Autodesk Inventor part; units mm, degrees
ref_plane "YZ Plane" through (0, 0, 0) normal (1, 0, 0) x (0, 1, 0)
ref_plane "XZ Plane" through (0, 0, 0) normal (0, 1, 0) x (-1, 0, 0)
ref_plane "XY Plane" through (0, 0, 0) normal (0, 0, 1) x (1, 0, 0)
sketch "Sketch1" plane through (0, 0, 0) normal (0, 0, 1) x (1, 0, 0)
  line L0 (-18.15, -21.15) -> (18.15, -21.15)
  line L1 (21.15, -18.15) -> (21.15, 18.15)
  line L2 (18.15, 21.15) -> (-18.15, 21.15)
  line L3 (-21.15, 18.15) -> (-21.15, -18.15)
  line L4 (-21.15, -21.15) -> (21.15, 21.15) construction
  line L5 (21.15, -21.15) -> (-21.15, 21.15) construction
  line L6 (-21.15, 18.15) -> (-18.15, 21.15)
  line L7 (18.15, 21.15) -> (21.15, 18.15)
  line L8 (21.15, -18.15) -> (18.15, -21.15)
  line L9 (-18.15, -21.15) -> (-21.15, -18.15)
  line L10 (-15.5, -15.5) -> (15.5, -15.5) construction
  line L11 (15.5, -15.5) -> (15.5, 15.5) construction
  line L12 (15.5, 15.5) -> (-15.5, 15.5) construction
  line L13 (-15.5, 15.5) -> (-15.5, -15.5) construction
  line L14 (-15.5, -15.5) -> (15.5, 15.5) construction
  line L15 (15.5, -15.5) -> (-15.5, 15.5) construction
  circle A0 centre (-15.5, 15.5) radius 1.5
  circle A1 centre (15.5, 15.5) radius 1.5
  circle A2 centre (15.5, -15.5) radius 1.5
  circle A3 centre (-15.5, -15.5) radius 1.5
  point P0 (0, 0)
  dimension "d0" = 42.3
  dimension "d1" = 42.3
  dimension "d2" = 3
  dimension "d3" = 3
  dimension "d4" = 3
  dimension "d5" = 3
  dimension "d6" = 3
  dimension "d7" = 3
  dimension "d8" = 3
  dimension "d9" = 3
  dimension "d10" = 31
  dimension "d11" = 31
  dimension "d12" = 3
  dimension "d13" = 3
  dimension "d14" = 3
  dimension "d15" = 3
extrude "Extrusion1" add sketch "Sketch1" along normal mid plane 48
sketch "Sketch2" plane through (0, 0, 0) normal (0, 0, 1) x (1, 0, 0)
  circle A0 centre (-15.5, 15.5) radius 1.5
  circle A1 centre (15.5, 15.5) radius 1.5
  circle A2 centre (15.5, -15.5) radius 1.5
  circle A3 centre (-15.5, -15.5) radius 1.5
  point P0 (0, 0)
extrude "Extrusion2" add sketch "Sketch2" along normal mid plane 40
sketch "Sketch3" plane through (0, 0, 0) normal (0, 0, 1) x (1, 0, 0)
  line L0 (10.8431, -20.5) -> (-10.8431, -20.5)
  line L1 (-20.5, -10.8431) -> (-20.5, 10.8431)
  line L2 (-10.8431, 20.5) -> (10.8431, 20.5)
  line L3 (20.5, 10.8431) -> (20.5, -10.8431)
  line L4 (20.5, -20.5) -> (-20.5, 20.5) construction
  line L5 (-20.5, -20.5) -> (20.5, 20.5) construction
  line L6 (-19.3284, 13.6716) -> (-13.6716, 19.3284)
  line L7 (13.6716, 19.3284) -> (19.3284, 13.6716)
  line L8 (19.3284, -13.6716) -> (13.6716, -19.3284)
  line L9 (-13.6716, -19.3284) -> (-19.3284, -13.6716)
  arc A0 (-10.8431, 20.5) -> (-13.6716, 19.3284) centre (-10.8431, 16.5) ccw
  arc A1 (-19.3284, 13.6716) -> (-20.5, 10.8431) centre (-16.5, 10.8431) ccw
  arc A2 (13.6716, 19.3284) -> (10.8431, 20.5) centre (10.8431, 16.5) ccw
  arc A3 (20.5, 10.8431) -> (19.3284, 13.6716) centre (16.5, 10.8431) ccw
  arc A4 (19.3284, -13.6716) -> (20.5, -10.8431) centre (16.5, -10.8431) ccw
  arc A5 (10.8431, -20.5) -> (13.6716, -19.3284) centre (10.8431, -16.5) ccw
  arc A6 (-13.6716, -19.3284) -> (-10.8431, -20.5) centre (-10.8431, -16.5) ccw
  arc A7 (-20.5, -10.8431) -> (-19.3284, -13.6716) centre (-16.5, -10.8431) ccw
  line L10 (-21.15, 18.15) -> (-18.15, 21.15)
  line L11 (-18.15, 21.15) -> (18.15, 21.15)
  line L12 (18.15, 21.15) -> (21.15, 18.15)
  line L13 (21.15, 18.15) -> (21.15, -18.15)
  line L14 (21.15, -18.15) -> (18.15, -21.15)
  line L15 (18.15, -21.15) -> (-18.15, -21.15)
  line L16 (-18.15, -21.15) -> (-21.15, -18.15)
  line L17 (-21.15, -18.15) -> (-21.15, 18.15)
  circle A8 centre (-15.5, 15.5) radius 1.5
  circle A9 centre (15.5, 15.5) radius 1.5
  circle A10 centre (15.5, -15.5) radius 1.5
  circle A11 centre (-15.5, -15.5) radius 1.5
  point P0 (0, 0)
  point P1 (-20.5, 12.5)
  point P2 (-12.5, 20.5)
  point P3 (12.5, 20.5)
  point P4 (20.5, 12.5)
  point P5 (20.5, -12.5)
  point P6 (12.5, -20.5)
  point P7 (-12.5, -20.5)
  point P8 (-20.5, -12.5)
  point P9 (-11.3431, -21.15)
  point P10 (-21.15, -11.4931)
  point P11 (11.3431, -21.15)
  point P12 (21.15, -11.4931)
  point P13 (21.15, 11.4931)
  point P14 (11.3431, 21.15)
  point P15 (-11.3431, 21.15)
  point P16 (-21.15, 11.4931)
  dimension "d20" = 41
  dimension "d21" = 41
  dimension "d22" = 8
  dimension "d23" = 8
  dimension "d24" = 8
  dimension "d25" = 8
  dimension "d26" = 8
  dimension "d27" = 8
  dimension "d28" = 8
  dimension "d29" = 8
  dimension "d30" = 4
extrude "Extrusion3" cut sketch "Sketch3" along normal mid plane 36 contours L8 A10 | A11 L9 | L7 A9 | A8 L6 | L10 L11 L12 L13 L14 L15 L16 L17 picked at (16.5579, -16.478) picked at (-16.478, -16.5579) picked at (16.5579, 16.478) picked at (-16.5579, 16.478)
sketch "Sketch4" plane through (0, 0, 24) normal (0, 0, 1) x (1, 0, 0)
  circle A0 centre (0, 0) radius 11
  dimension "d33" = 22
extrude "Extrusion4" add sketch "Sketch4" along normal blind 2
sketch "Sketch5" plane through (0, 0, 26) normal (0, 0, 1) x (1, 0, 0)
  circle A0 centre (0, 0) radius 2.5
  dimension "d36" = 5
extrude "Extrusion5" add sketch "Sketch5" along normal blind 22
sketch "Sketch6" plane through (0, 0, 26) normal (0, 0, 1) x (1, 0, 0)
  circle A0 centre (0, 0) radius 2.5
  circle A1 centre (0, 0) radius 4.5
  dimension "d39" = 2
extrude "Extrusion6" cut sketch "Sketch6" against normal blind 2
fillet "Fillet1" radius 1 3 edges at (-11, 0, 24) (-4.5, 0, 26) (-11, 0, 26)
equation "\"d3\" = d2"
equation "\"d4\" = d2"
equation "\"d5\" = d4"
equation "\"d6\" = d2"
equation "\"d7\" = d6"
equation "\"d8\" = d2"
equation "\"d9\" = d8"
properties part number "3217_Stepper Motor_V1" material "Stainless Steel, Brushed"
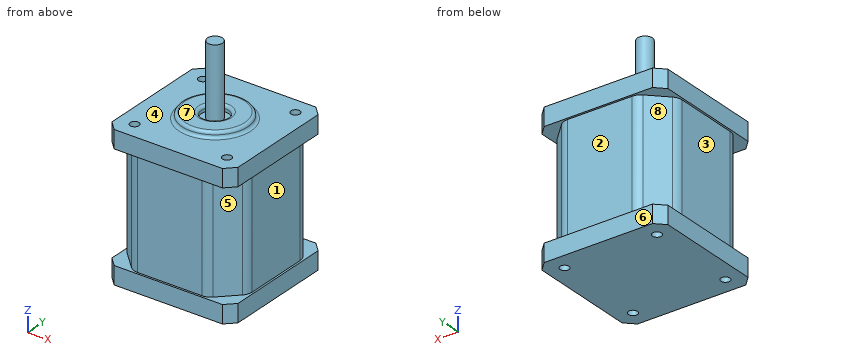
Verification items for the finished model (mm, model axes). Face numbers are marked on the shaded views. A direction names the side the tool comes from. Coordinates: 2 decimals unless noted, no trailing zeros. Order: outer loops, then holes, each group sorted by start corner. A loop starts at its lowest first (then second) coordinate and runs counter-clockwise, first axis right, second up. Notation, with made-up numbers: (26.25, 3) -> (54.25, 3) arc R19 ccw to (54.25, 31) -> close; hole circle Ø11 at (2.5, 1.25). An arc over 180 degrees is marked (long way). Put each result on its own line as item: value. Start each with the question number.
1) Material ranges on L1, parallel to Y at x = -15.5, z = 22; L2, parallel to Y at x = -15, z = 21; L3, parallel to X at y = -4, z = 6.5, recorded low to high.
2) Cross-section at A-A (y = -15.5). Enter the section's corners in (x, z).
3) Release check for a two-part mould opening along Z. For the marked faces 6, 7 and 8 record: pulls with the +Z half, pulls with the -Z half, needs draft (parallel to the pull), parting line crosses it, or undercut.
4) Cross-section at C-C (z = -1.5). Enter the section's corners in (x, y), plus the area to 3 significant figures.
5) Go/stop test with flat-tipped pins: pin 1 (3.5 mm diameter, centred on x = -16, y = -16, fed in from -Z); pin 2 (2.5 mm diameter, centred on x = -15.5, y = -15.5, fed in from +Z); pin 3 (2.5 mm diameter, centred on x = 15.5, y = -15.5, fed in from -Z); pin 4 (10 mm diameter, centred on x = 6, y = -12.5, fed in from +Z). Record where each tip stops, or that it passes through.
6) Tool access check on the marked faces 1, 2, 3, 4 and 5. Record the directions out of +Z, -Z, +X, -X, +Y, -Y that give a thin tool (end or side, any length) a straight path to the whole face; none if there is none.
Geometry check:
1. L1: y = -21.15 to -17, -14 to 14, 17 to 21.15
1. L2: y = -21.15 to -16.91, -14.09 to 14.09, 16.91 to 21.15
1. L3: x = -20.5 to 20.5
2. outline: (-21.15, -24) -> (-17, -24) -> (-17, -20) -> (-14, -20) -> (-14, -24) -> (14, -24) -> (14, -20) -> (17, -20) -> (17, -24) -> (21.15, -24) -> (21.15, -18) -> (17.5, -18) -> (17.5, 18) -> (21.15, 18) -> (21.15, 24) -> (17, 24) -> (17, 20) -> (14, 20) -> (14, 24) -> (-14, 24) -> (-14, 20) -> (-17, 20) -> (-17, 24) -> (-21.15, 24) -> (-21.15, 18) -> (-17.5, 18) -> (-17.5, -18) -> (-21.15, -18) -> close
3. face 6: needs draft
3. face 7: pulls with the +Z half
3. face 8: undercut
4. outline: (-20.5, -10.84) arc R4 ccw to (-19.33, -13.67) -> (-13.67, -19.33) arc R4 ccw to (-10.84, -20.5) -> (10.84, -20.5) arc R4 ccw to (13.67, -19.33) -> (19.33, -13.67) arc R4 ccw to (20.5, -10.84) -> (20.5, 10.84) arc R4 ccw to (19.33, 13.67) -> (13.67, 19.33) arc R4 ccw to (10.84, 20.5) -> (-10.84, 20.5) arc R4 ccw to (-13.67, 19.33) -> (-19.33, 13.67) arc R4 ccw to (-20.5, 10.84) -> close
4. area: 1,550 mm^2
5. pin 1: stops at z = -24
5. pin 2: stops at z = 20
5. pin 3: stops at z = -20
5. pin 4: stops at z = 26
6. face 1: +X, +Y, -Y
6. face 2: +X, -X, +Y
6. face 3: -X, +Y, -Y
6. face 4: +Z
6. face 5: +X, -Y
